```python
from build123d import *

# Parameters (mm, degrees)
F0_W     = 76.2
F0_H     = 127
F1_DEPTH = 12.7
F2_T     = -7.62
F4_DEPTH = 63.5


with BuildPart() as f1:
    # F0 (on Top) → F1 (new body)
    with BuildSketch(Plane.XY):
        Rectangle(F0_W, F0_H)
    extrude(amount=F1_DEPTH)

    # F2
    f2_openings = [f1.faces().sort_by_distance(p)[0] for p in [
        (0, 0, 12.7),
    ]]
    offset(amount=F2_T, openings=f2_openings)

    # F3 (on Front) → F4 (join, symmetric)
    with BuildSketch(Plane.XZ):
        Polygon((-38.1, 4.947344), (-39.625825, 4.947344), (-39.625825, 2.672656), (-38.1, 2.672656), (-38.1, 3.81), align=None)
        Polygon((-39.625825, 2.672656), (-39.625825, 4.947344), (-39.625825, 6.35), (-40.895825, 6.35), (-40.895825, 1.27), (-39.625825, 1.27), align=None)
        Polygon((39.625825, 6.35), (39.625825, 4.947344), (39.625825, 2.672656), (39.625825, 1.27), (40.895825, 1.27), (40.895825, 6.35), align=None)
        Polygon((39.625825, 2.672656), (39.625825, 4.947344), (38.1, 4.947344), (38.1, 3.81), (38.1, 2.672656), align=None)
    extrude(amount=F4_DEPTH, both=True)


solid = f1.part
```
Part model, mm, in its own coordinate system. A direction names the side the tool comes from. Give positions to 0.01 mm unless a question says otherwise; leave off trailing zeros. Write each loop counter-clockwise with the first axis right and the second up, starting at its lowest first coordinate (ties: lowest second). Pieces come first, ordered by that corner, then holes. Notation, with made-up numbers: (62, 18.25) -> (115, 18.25) arc R25 cw to (115, 45.25) -> close; hole circle Ø3 at (64, 34.25). An arc over 180 degrees is marked (long way). Put each result on its own line as item: value. Start each with the question number.
Item 1: Cut at B-B (y = -38). List the corners of the cut face in (x, z).
Item 2: Wall check: L1, parallel to X at y = 35, z = 5.5; L2, parallel to Y at x = -22, z = 9; L3, parallel to X at y = 35, z = 12. Give the ranges that are in metal, low to high. Write a range as [from, to].
Item 3: Pull direction Y, two halves, no side cores. Call faces 5 (the face through (-38.1, -1, 9)), 6 (the face through (-1, 63.5, 6)), 7 (the face through (-30.48, -1, 10)): pulls with the +Y half, pulls with the -Y half, needs draft (parallel to the pull), parting line crosses it, or undercut.
Item 4: Cut at A-A (z = 9). List the corners of the cut face in (x, y).
Item 5: Which spindle directions (+Z, -Z, +X, -X, +Y, -Y) get a long thin tool onto all of the face, cutting with end or side? Do faces 1 (the face through (38.1, -1, 9)), 2 (the face through (40.896, -1, 4)), 3 (the face through (-38.1, -1, 1)), 4 (the face through (0, 55.88, 10)). Say none if no direction does.
Item 6: Pin check, flat tips, straight feed: pin 1 Ø0.8 at (x, y) = (-39, 15.5) entering from -Z; pin 2 Ø5.5 at (y, z) = (14.5, 10.5) entering from +X; pin 3 Ø1 at (x, y) = (40, -11.5) entering from +Z. Stop position of each tip, or through.
Item 7: Cut at C-C (x = -21). List the corners of the cut face in (y, z), then the cut area to 3 significant figures.
Answer list:
1. outline: (-40.9, 1.27) -> (-39.63, 1.27) -> (-39.63, 2.67) -> (-38.1, 2.67) -> (-38.1, 0) -> (38.1, 0) -> (38.1, 2.67) -> (39.63, 2.67) -> (39.63, 1.27) -> (40.9, 1.27) -> (40.9, 6.35) -> (39.63, 6.35) -> (39.63, 4.95) -> (38.1, 4.95) -> (38.1, 12.7) -> (30.48, 12.7) -> (30.48, 7.62) -> (-30.48, 7.62) -> (-30.48, 12.7) -> (-38.1, 12.7) -> (-38.1, 4.95) -> (-39.63, 4.95) -> (-39.63, 6.35) -> (-40.9, 6.35) -> close
2. L1: x = [-40.9, -39.63], [-38.1, 38.1], [39.63, 40.9]
2. L2: y = [-63.5, -55.88], [55.88, 63.5]
2. L3: x = [-38.1, -30.48], [30.48, 38.1]
3. face 5: needs draft
3. face 6: pulls with the +Y half
3. face 7: undercut
4. outline: (-38.1, -63.5) -> (38.1, -63.5) -> (38.1, 63.5) -> (-38.1, 63.5) -> close; hole (-30.48, -55.88) -> (30.48, -55.88) -> (30.48, 55.88) -> (-30.48, 55.88) -> close
5. face 1: +Z, +Y, -Y
5. face 2: +Z, -Z, +X, +Y, -Y
5. face 3: -Z, +Y, -Y
5. face 4: +Z
6. pin 1: stops at z = 2.67
6. pin 2: stops at x = 38.1
6. pin 3: stops at z = 6.35
7. outline: (-63.5, 0) -> (63.5, 0) -> (63.5, 12.7) -> (55.88, 12.7) -> (55.88, 7.62) -> (-55.88, 7.62) -> (-55.88, 12.7) -> (-63.5, 12.7) -> close
7. area: 1,050 mm2
